Part print with two shaded views. Sizes in mm from the minimum x, y, z corner. A direction names the side the tool comes from. Round coordinates to 2 decimals unless told otherwise and drop trailing zeros. Loops run counter-clockwise (first coordinate to the right, second up) from the corner with the lowest first, then second, coordinate; pieces in that order, holes last.
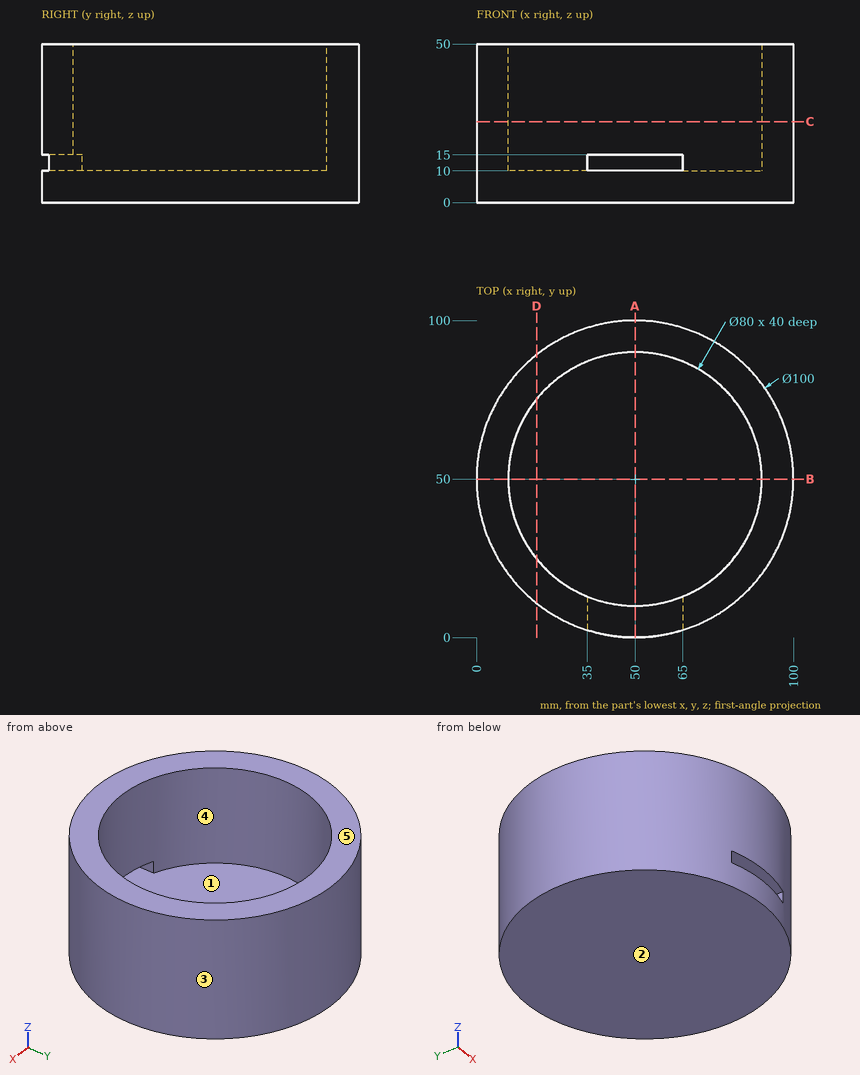
Item 1: Mould opens along Y. For the marked faces 1, 2 and 3 say: released by +Y, released by -Y, zero draft, split by the parting line, or undercut.
Verdict:
face 1: undercut
face 2: zero draft
face 3: split by the parting line
Item 2: Cut at C-C (z = 25.5). List the corners of the cut face in (x, y).
Verdict:
outline: circle Ø100 at (50, 50); hole circle Ø80 at (50, 50)
Item 3: Wall check: L1, parallel to Y at x = 50, z = 22; L2, parallel to Y at x = 22.5, z = 17.5; L3, parallel to X at y = 55, z = 16. Give the ranges that are in metal, low to high.
Verdict:
L1: y = 0 to 10, 90 to 100
L2: y = 8.24 to 20.95, 79.05 to 91.76
L3: x = 0.25 to 10.31, 89.69 to 99.75
Item 4: Cut at D-D (x = 19). List the corners of the cut face in (y, z), plus the area to 3 significant figures.
Verdict:
outline: (10.77, 0) - (89.23, 0) - (89.23, 50) - (75.28, 50) - (75.28, 10) - (24.72, 10) - (24.72, 50) - (10.77, 50) - close
area: 1,900 mm2
Item 5: Cut at A-A (x = 50). List the corners of the cut face in (y, z).
Verdict:
outline: (0, 0) - (100, 0) - (100, 50) - (90, 50) - (90, 10) - (0, 10) - close; (0, 15) - (10, 15) - (10, 50) - (0, 50) - close
Item 6: 3-axis set-ups, long thin cutter, end or side, ignore diameter. For the marked faces 4 and 5: which of +Z, -Z, +X, -X, +Y, -Y reach the whole face in a straight line?
Verdict:
face 4: +Z
face 5: +Z, +X, -X, +Y, -Y
Item 7: Flat gauge pins, fed straight in: P1, Ø2.5, axis at y = 9, z = 12, coming from the +X side; P2, Ø1, axis at y = 88, z = 37, coming from the +X side; P3, Ø4, axis at y = 39.5, z = 15, coming from the -X side; P4, Ø14, axis at x = 46, y = 5, coming from the -Z side. Where does each tip first touch, or does it go through?
Verdict:
P1: stops at x = 80.33
P2: stops at x = 83.07
P3: stops at x = 0.73
P4: stops at z = 0
Item 8: Cut at B-B (y = 50). List the corners of the cut face in (x, z), plus the area to 3 significant figures.
Verdict:
outline: (0, 0) - (100, 0) - (100, 50) - (90, 50) - (90, 10) - (10, 10) - (10, 50) - (0, 50) - close
area: 1,800 mm2
